from build123d import *

# Parameters (mm, degrees)
F0_R     = 1.6
F1_DEPTH = 5
F2_W     = 29.5
F2_H     = 5
F3_DEPTH = 10
F4_W     = 29.5
F4_H     = 15
F5_DEPTH = 4
F6_R     = 2.25
F7_DEPTH = 25
F8_W     = 23.5
F8_H     = 5.420308
F9_DEPTH = 25


with BuildPart() as f1:
    # F0 (on Top) → F1 (new body)
    with BuildSketch(Plane.XY):
        with BuildLine():
            Line((14.75, 6.5), (-14.75, 6.5))
            Line((-14.75, 6.5), (-14.75, 3.725468))
            Line((-14.75, 3.725468), (-14.75, -3.75))
            Line((-14.75, -3.75), (-14.75, -6.5))
            Line((-14.75, -6.5), (14.75, -6.5))
            Line((14.75, -6.5), (14.75, -3.75))
            Line((14.75, -3.75), (18.5, -3.75))
            ThreePointArc((18.5, -3.75), (22.25, 0), (18.5, 3.75))
            Line((18.5, 3.75), (14.75, 3.75))
            Line((14.75, 3.75), (14.75, 6.5))
        make_face()
        with Locations((18.5, 0)):
            Circle(F0_R, mode=Mode.SUBTRACT)
        with BuildLine():
            Line((-14.75, -3.75), (-14.75, 3.725468))
            Line((-14.75, 3.725468), (-18.475388, 3.749919))
            ThreePointArc((-18.475388, 3.749919), (-22.24998, 0.012306), (-18.5, -3.75))
            Line((-18.5, -3.75), (-14.75, -3.75))
        make_face()
        with Locations((-18.5, 0)):
            Circle(F0_R, mode=Mode.SUBTRACT)
    extrude(amount=F1_DEPTH)

    # F2 (on face) → F3 (join)
    with BuildSketch(Plane.XZ.offset(6.5)):
        with Locations((0, 2.5)):
            Rectangle(F2_W, F2_H)
    extrude(amount=F3_DEPTH)

    # F4 (on face) → F5 (join)
    with BuildSketch(Plane.XZ.offset(16.5)):
        with Locations((0, -2.5)):
            Rectangle(F4_W, F4_H)
    extrude(amount=F5_DEPTH)

    # F6 (on face) → F7 (cut)
    with BuildSketch(Plane(origin=(0, -16.5, 0), x_dir=(-1, 0, 0), z_dir=(0, 1, 0))):
        with Locations((-9.75, -5)):
            Circle(F6_R)
        with Locations((9.75, -5)):
            Circle(F6_R)
    extrude(amount=-F7_DEPTH, mode=Mode.SUBTRACT)

    # F8 (on face) → F9 (cut)
    with BuildSketch(Plane(origin=(0, 0, 0), x_dir=(1, 0, 0), z_dir=(0, 0, -1))):
        with Locations((0, 9.210154)):
            Rectangle(F8_W, F8_H)
    extrude(amount=-F9_DEPTH, mode=Mode.SUBTRACT)


solid = f1.part
Source: CAD feature listing. Evaluate the final solid. Frame: model axes, mm. A direction names the side the tool comes from. Give positions to 0.01 mm unless a question says otherwise; leave off trailing zeros. Order: outer loops, then holes, each group sorted by start corner. A loop starts at its lowest first (then second) coordinate and runs counter-clockwise, first axis right, second up. Notation, with made-up numbers: (-11, 77) -> (38, 77) arc R11 ccw to (38, 92) -> close; hole circle Ø3 at (65, 61). An arc over 180 degrees is marked (long way). Use a Markdown table: item, result.
1) Ray query, line 1 along Z through (x, y) = (-9.75, -18.1); line 2 along X through (y, z) = (-18, -4); line 3 along Y through (x, z) = (-10.5, 1.25). Return the intervals inside material, ascending. Write a range as [from, to].
Answer list:
| item | result |
|---|---|
| line 1 | [-10, -7.25], [-2.75, 5] |
| line 2 | [-14.75, -11.77], [-7.73, 7.73], [11.77, 14.75] |
| line 3 | [-20.5, -11.92], [-6.5, 6.5] |
2) Contact query for flat-ended pins moving along their axis: P1, Ø3, axis at x = -17.5, z = 3, coming from the -Y side; P2, Ø2, axis at y = 5.5, z = 2, coming from the -X side; P3, Ø8, axis at y = -17.5, z = 0.5, coming from the +X side. Output: stop coordinate, or through.
Answer list:
| item | result |
|---|---|
| P1 | y = -3.75 |
| P2 | x = -14.75 |
| P3 | x = 14.75 |
3) Mould query, pull axis Y, two halves, no side actions, for faces 6 (the flat face through (0, -16.5, -5)), 7 (the cylindrical face through (-20.1, 0.07, 2.46)), 8 (the flat face through (11.75, -9, 2)), 9 (the flat face through (14.75, 5, 2)). Classes: +Y half, -Y half, draft (parallel to the pull), parting line (faces both ways), or undercut.
Answer list:
| item | result |
|---|---|
| face 6 | +Y half |
| face 7 | undercut |
| face 8 | undercut |
| face 9 | draft |
4) Reachability of faces 1 (the flat face through (-14.75, -14, 1)), 2 (the flat face through (-11.75, -9, 2)), 3 (the flat face through (0, -2, 0)), 4 (the flat face through (17, 3.75, 2)), 5 (the flat face through (17, -3.75, 2)) from +Z, -Z, +X, -X, +Y, -Y: full face, straight path, thin tool, end or side. Return the list, or none.
Answer list:
| item | result |
|---|---|
| face 1 | +Z, -Z, -X, -Y |
| face 2 | +Z, -Z |
| face 3 | -Z, +X, -X, +Y |
| face 4 | +Z, -Z, +X, +Y |
| face 5 | +Z, -Z, +X, -Y |
5) Section query D-D, the plane z = -5. Return the cut outline in (x, y).
Answer list:
| item | result |
|---|---|
| outline | (-14.75, -20.5) -> (-12, -20.5) -> (-12, -16.5) -> (-14.75, -16.5) -> close; (-7.5, -20.5) -> (7.5, -20.5) -> (7.5, -16.5) -> (-7.5, -16.5) -> close; (12, -20.5) -> (14.75, -20.5) -> (14.75, -16.5) -> (12, -16.5) -> close |
6) Section query B-B, the plane z = 4. Return the cut outline in (x, y).
Answer list:
| item | result |
|---|---|
| outline | (-18.5, -3.75) -> (-14.75, -3.75) -> (-14.75, -20.5) -> (14.75, -20.5) -> (14.75, -3.75) -> (18.5, -3.75) arc R3.75 ccw to (18.5, 3.75) -> (14.75, 3.75) -> (14.75, 6.5) -> (-14.75, 6.5) -> (-14.75, 3.73) -> (-18.48, 3.75) arc R3.75 ccw (long way) to start; hole circle Ø3.2 at (-18.5, 0); hole (-11.75, -11.92) -> (11.75, -11.92) -> (11.75, -6.5) -> (-11.75, -6.5) -> close; hole circle Ø3.2 at (18.5, 0) |
7) Section query A-A, the plane y = -10. Return the cut outline in (x, z), then the cut area to 3 significant figures.
Answer list:
| item | result |
|---|---|
| outline | (-14.75, 0) -> (-11.75, 0) -> (-11.75, 5) -> (-14.75, 5) -> close; (11.75, 0) -> (14.75, 0) -> (14.75, 5) -> (11.75, 5) -> close |
| area | 30.0 mm² |
8) Section query C-C, the plane x = 9.75. Return the cut outline in (y, z), then the cut area to 3 significant figures.
Answer list:
| item | result |
|---|---|
| outline | (-20.5, -10) -> (-16.5, -10) -> (-16.5, -7.25) -> (-20.5, -7.25) -> close; (-20.5, -2.75) -> (-16.5, -2.75) -> (-16.5, 0) -> (-11.92, 0) -> (-11.92, 5) -> (-20.5, 5) -> close; (-6.5, 0) -> (6.5, 0) -> (6.5, 5) -> (-6.5, 5) -> close |
| area | 130 mm² |
